Input: part model. Units: mm. Frame: model coordinates. A direction names the side the tool comes from. Coordinates: 2 decimals unless noted, no trailing zeros. Write each loop counter-clockwise with the first axis right and the second up, starting at its lowest first coordinate (ties: lowest second). Pieces come first, ordered by that corner, then holes. Notation, with made-up numbers: M 41.25,34 L 54.25,34 A24 ccw 54.25,68 Z; hole C 80.5,71.25 d3. An arc over 180 degrees is marked long. Use one line per item in the form item = value.
from build123d import *

# Parameters (mm, degrees)
BOSS_EXTRUDE1_DEPTH      = 10
BOSS_EXTRUDE1_DEPTH_BACK = 28
SKETCH1_W                = 40
SKETCH1_H                = 20
SKETCH2_R                = 2.5
BOSS_EXTRUDE2_DEPTH      = 8
SKETCH3_W                = 7.25
SKETCH3_H                = 18
BOSS_EXTRUDE3_DEPTH      = 2.5
SKETCH4_R                = 2.25
CUT_EXTRUDE1_DEPTH       = 44.866388044


with BuildPart() as part:
    # Sketch1 → Boss-Extrude1 (new, two sides: drawn at the far end of the back side and taken through both)
    with BuildSketch(Plane(origin=(0, 0, 0), x_dir=(1, 0, 0), z_dir=(0, 1, 0)).offset(-BOSS_EXTRUDE1_DEPTH_BACK)):
        with Locations((-9.9, 0)):
            Rectangle(SKETCH1_W, SKETCH1_H)
    extrude(amount=BOSS_EXTRUDE1_DEPTH + BOSS_EXTRUDE1_DEPTH_BACK)

    # Sketch2 → Boss-Extrude2 (add)
    with BuildSketch(Plane(origin=(0, 10, 0), x_dir=(1, 0, 0), z_dir=(0, 1, 0))):
        with Locations(Location((0, 0, 0), (0, 0, 270))):
            Circle(SKETCH2_R)
    extrude(amount=BOSS_EXTRUDE2_DEPTH)

    # Sketch3 → Boss-Extrude3 (add)
    with BuildSketch(Plane(origin=(0, 0, 0), x_dir=(1, 0, 0), z_dir=(0, 1, 0))):
        with Locations((13.725, 0)):
            Rectangle(SKETCH3_W, SKETCH3_H)
    boss_extrude3 = extrude(amount=BOSS_EXTRUDE3_DEPTH)

    # Sketch4 → Cut-Extrude1 (cut, symmetric)
    with BuildSketch(Plane(origin=(0, 2.5, 0), x_dir=(1, 0, 0), z_dir=(0, 1, 0))):
        with Locations(Location((14.85, -5, 0), (0, 0, 270))):
            Circle(SKETCH4_R)
        with Locations(Location((14.85, 5, 0), (0, 0, 270))):
            Circle(SKETCH4_R)
    cut_extrude1 = extrude(amount=CUT_EXTRUDE1_DEPTH, both=True, mode=Mode.SUBTRACT)

    # Mirror1: Boss-Extrude3, Cut-Extrude1 across plane
    add(boss_extrude3.mirror(Plane.ZY.offset(9.9)))
    add(cut_extrude1.mirror(Plane.ZY.offset(9.9)), mode=Mode.SUBTRACT)


solid = part.part
(1) First-contact query: pin 1 Ø8 at (y, z) = (12, -6) entering from +X; pin 2 Ø0.8 at (x, y) = (12, 1.5) entering from -Z; pin 3 Ø7 at (x, z) = (14.85, -5) entering from +Y; pin 4 Ø4 at (x, z) = (14.85, 5) entering from -Y. Flat tips, straight axial feed; report the tip coordinate or a pass-through.
Computed:
pin_1 = 10.1
pin_2 = -9
pin_3 = 2.5
pin_4 = through
(2) Section query D-D on z = 5.25. Return the cut outline in (x, y).
Computed:
outline = M -37.15,0 L -36.89,0 L -36.89,2.5 L -37.15,2.5 Z; M -32.41,0 L -29.9,0 L -29.9,-28 L 10.1,-28 L 10.1,0 L 12.61,0 L 12.61,2.5 L 10.1,2.5 L 10.1,10 L -29.9,10 L -29.9,2.5 L -32.41,2.5 Z; M 17.09,0 L 17.35,0 L 17.35,2.5 L 17.09,2.5 Z
(3) Set-up query: faces 1 (the flat face through (-33, 2.5, 0)), 2 (the flat face through (14, 2.5, 0)), 3 (the flat face through (14, 1, -9)), 4 (the flat face through (-33, 1, -9)), 5 (the flat face through (-33, 1, 9)). Return all of +Z, -Z, +X, -X, +Y, -Y with unobstructed straight access to the full face (end or side cutting, diameter ignored); none if empty.
Computed:
face_1 = +Z, -Z, -X, +Y
face_2 = +Z, -Z, +X, +Y
face_3 = -Z, +X, +Y, -Y
face_4 = -Z, -X, +Y, -Y
face_5 = +Z, -X, +Y, -Y
(4) Section query B-B on z = -5. Return the cut outline in (x, y).
Computed:
outline = M -37.15,0 L -36.9,0 L -36.9,2.5 L -37.15,2.5 Z; M -32.4,0 L -29.9,0 L -29.9,-28 L 10.1,-28 L 10.1,0 L 12.6,0 L 12.6,2.5 L 10.1,2.5 L 10.1,10 L -29.9,10 L -29.9,2.5 L -32.4,2.5 Z; M 17.1,0 L 17.35,0 L 17.35,2.5 L 17.1,2.5 Z
(5) Pull-direction query (Z, two-part tool) for faces 6 (the cylindrical face through (-2.44, 13.94, -0.54)), 7 (the flat face through (17.35, 1, 0)), 8 (the cylindrical face through (-32.654, 1.268, -3.962)); classes: pulls with the +Z half, pulls with the -Z half, needs draft (parallel to the pull), parting line crosses it, or undercut.
Computed:
face_6 = parting line crosses it
face_7 = needs draft
face_8 = undercut
(6) Section query A-A on x = -34.65. Return the cut outline in (y, z).
Computed:
outline = M 0,-9 L 2.5,-9 L 2.5,-7.25 L 0,-7.25 Z; M 0,-2.75 L 2.5,-2.75 L 2.5,2.75 L 0,2.75 Z; M 0,7.25 L 2.5,7.25 L 2.5,9 L 0,9 Z
(7) Section query C-C on z = 0. Return the cut outline in (x, y).
Computed:
outline = M -37.15,0 L -29.9,0 L -29.9,-28 L 10.1,-28 L 10.1,0 L 17.35,0 L 17.35,2.5 L 10.1,2.5 L 10.1,10 L 2.5,10 L 2.5,18 L -2.5,18 L -2.5,10 L -29.9,10 L -29.9,2.5 L -37.15,2.5 Z
(8) Line query: probe 1 along X at (y, z) = (1.7, -5); probe 2 along X at (y, z) = (-9, -5.75); probe 3 along Z at (x, y) = (-34, 1). Output: solid intervals per line, ascending.
Computed:
probe_1 = -37.15 to -36.9, -32.4 to 12.6, 17.1 to 17.35
probe_2 = -29.9 to 10.1
probe_3 = -9 to -7.15, -2.85 to 2.85, 7.15 to 9
